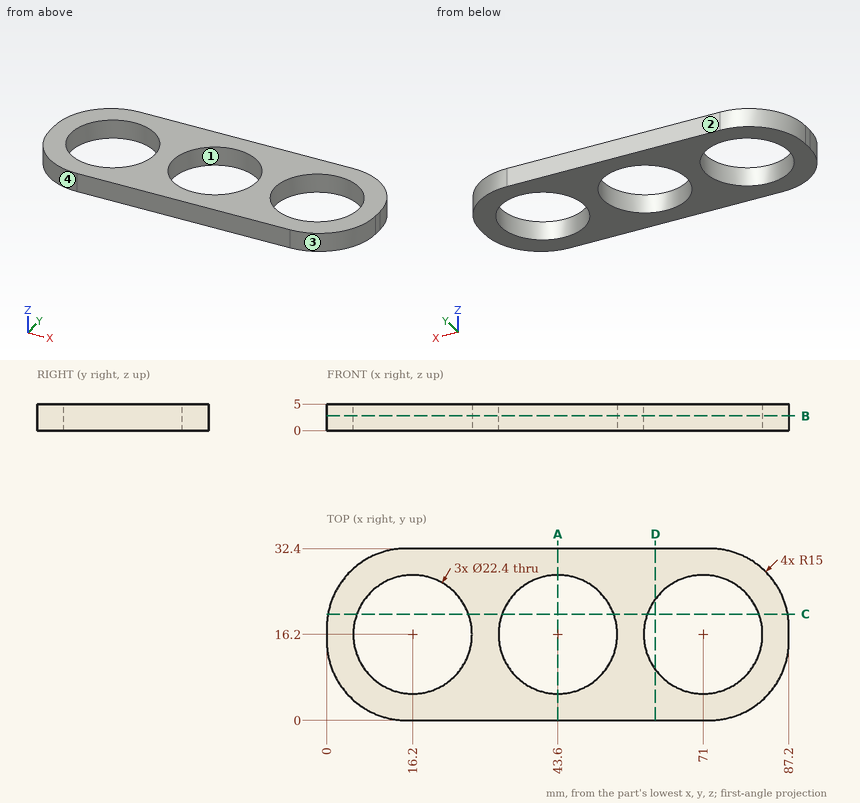
Input: dimensioned drawing with shaded views. Units: mm. Origin: part minimum x, y, z. Give positions to 0.01 mm unless a question says otherwise; leave off trailing zeros. Write each loop counter-clockwise with the first axis right and the second up, starting at its lowest first coordinate (ties: lowest second). Pieces come first, ordered by that corner, then holes.
Q1. Section D-D, the plane x = 62. Output: boundary loops of the cut face in (y, z).
Q2. Material intervals for probe 1 along Y at (x, z) = (71, 1); probe 2 along X at (y, z) = (11.5, 3.3); probe 3 along X at (y, z) = (10, 3.45), sorted ascending.
Q3. Section A-A, the plane x = 43.6. Output: boundary loops of the cut face in (y, z), plus the area to 3 significant figures.
Q4. Pull-direction query (X, two-part tool) for the marked faces 1, 2, 3 and 4; classes: pulls with the +X half, pulls with the -X half, needs draft (parallel to the pull), parting line crosses it, or undercut.
Q5. First-contact query: P1, Ø1, axis at y = 3.5, z = 4.5, coming from the +X side. Flat tip, straight axial feed; report the tip coordinate or a pass-through.
Q6. Section C-C, the plane y = 20. Output: boundary loops of the cut face in (x, z), plus the area to 3 significant figures.
Q7. Section B-B, the plane z = 2.75. Output: boundary loops of the cut face in (x, y), plus the area to 3 significant figures.
Filled in:
1. outline: (0, 0) - (9.53, 0) - (9.53, 5) - (0, 5) - close; (22.87, 0) - (32.4, 0) - (32.4, 5) - (22.87, 5) - close
2. probe 1: y = 0 to 5, 27.4 to 32.4
2. probe 2: x = 0.41 to 6.03, 26.37 to 33.43, 53.77 to 60.83, 81.17 to 86.79
2. probe 3: x = 0.86 to 6.87, 25.53 to 34.27, 52.93 to 61.67, 80.33 to 86.34
3. outline: (0, 0) - (5, 0) - (5, 5) - (0, 5) - close; (27.4, 0) - (32.4, 0) - (32.4, 5) - (27.4, 5) - close
3. area: 50.0 mm2
4. face 1: undercut
4. face 2: needs draft
4. face 3: pulls with the +X half
4. face 4: pulls with the -X half
5. P1: stops at x = 82.4
6. outline: (0.23, 0) - (5.66, 0) - (5.66, 5) - (0.23, 5) - close; (26.74, 0) - (33.06, 0) - (33.06, 5) - (26.74, 5) - close; (54.14, 0) - (60.46, 0) - (60.46, 5) - (54.14, 5) - close; (81.54, 0) - (86.97, 0) - (86.97, 5) - (81.54, 5) - close
6. area: 118 mm2
7. outline: (0, 15) arc R15 ccw to (15, 0) - (72.2, 0) arc R15 ccw to (87.2, 15) - (87.2, 17.4) arc R15 ccw to (72.2, 32.4) - (15, 32.4) arc R15 ccw to (0, 17.4) - close; hole circle Ø22.4 at (16.2, 16.2); hole circle Ø22.4 at (43.6, 16.2); hole circle Ø22.4 at (71, 16.2)
7. area: 1,450 mm2
